Part print with two shaded views. Sizes in mm from the minimum x, y, z corner. A direction names the side the tool comes from. Coordinates: 2 decimals unless noted, no trailing zeros. Loops run counter-clockwise (first coordinate to the right, second up) from the corner with the lowest first, then second, coordinate; pieces in that order, holes last.
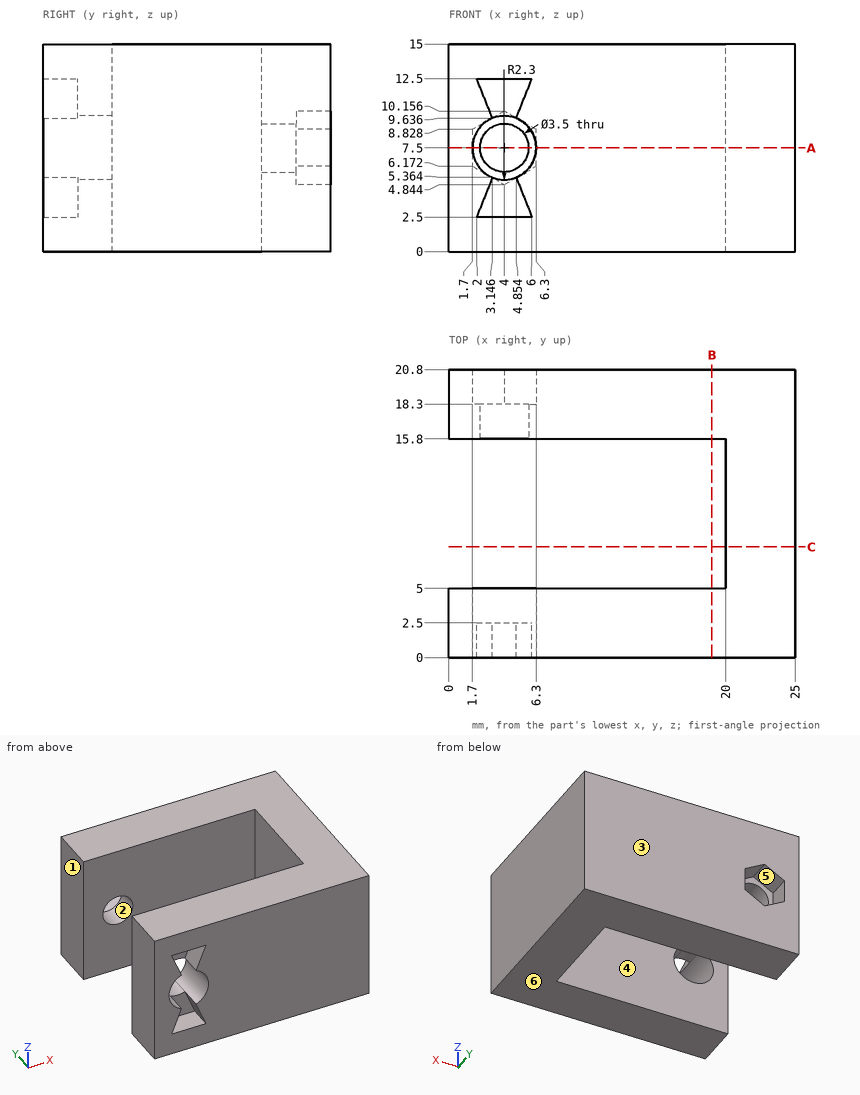
Q1. Slice it at A-A (z = 7.5). List the corners of the cut face in (x, y).
Answers:
outline: (0, 0) - (1.7, 0) - (1.7, 5) - (0, 5) - close; (0, 15.8) - (2.25, 15.8) - (2.25, 18.3) - (1.7, 18.3) - (1.7, 20.8) - (0, 20.8) - close; (5.75, 15.8) - (20, 15.8) - (20, 5) - (6.3, 5) - (6.3, 0) - (25, 0) - (25, 20.8) - (6.3, 20.8) - (6.3, 18.3) - (5.75, 18.3) - close
Q2. Slice it at B-B (x = 19). List the corners of the cut face in (y, z), and give its area (3 significant figures).
Answers:
outline: (0, 0) - (5, 0) - (5, 15) - (0, 15) - close; (15.8, 0) - (20.8, 0) - (20.8, 15) - (15.8, 15) - close
area: 150 mm2
Q3. Drill centre lines: line 1 (Z direction, x = 4, y = 16.65); line 2 (Y direction, x = 19, z = 14); line 3 (Z direction, x = 4.5, y = 1). Where is each one in solid material? Low to high.
Answers:
line 1: z = 0 to 5.75, 9.25 to 15
line 2: y = 0 to 5, 15.8 to 20.8
line 3: z = 0 to 2.5, 12.5 to 15
Q4. Which spindle directions (+Z, -Z, +X, -X, +Y, -Y) get a long thin tool onto all of the face, cutting with end or side? Do the marked faces 4, 5 and 6. Say none if no direction does.
Answers:
face 4: +Z, -Z, -X
face 5: +Y
face 6: -Z, +X, -X, +Y, -Y
Q5. Mould opens along X. For the marked faces 1, 2 and 3 say: +X half, -X half, draft (parallel to the pull), parting line (faces both ways), or undercut.
Answers:
face 1: -X half
face 2: undercut
face 3: draft
Q6. Slice it at C-C (y = 8). List the corners of the cut face in (x, z), and give its area (3 significant figures).
Answers:
outline: (20, 0) - (25, 0) - (25, 15) - (20, 15) - close
area: 75.0 mm2
Q7. Flat gauge pins, fed straight in: P1, Ø4, axis at y = 8, z = 8.5, coming from the -X side; P2, Ø1.4, axis at x = 4.5, z = 3.5, coming from the -Y side. Where does each tip first touch, or does it go through?
Answers:
P1: stops at x = 20
P2: stops at y = 2.5
